Design review of the part built by this model. Coordinates are the model's own, in mm. Face numbers are marked on the shaded views. Give positions to 0.01 mm unless a question says otherwise; leave off trailing zeros. Order: outer loops, then holes, each group sorted by start corner. A loop starts at its lowest first (then second) coordinate and runs counter-clockwise, first axis right, second up. Notation, with made-up numbers: (40.5, 25) -> (66.5, 25) arc R10 ccw to (66.5, 35) -> close; hole circle Ø10 at (84, 77). An arc over 180 degrees is marked (long way). One line per item, written item: value. Start each with the question number.
1) Consider section C-C (y = 4.2). State how many separate pieces and enclosed holes the cut face has, plus the area to 3 significant figures.
2) For pin 1 (1.6 mm diameter, centred on y = 2, z = 9.5, fed in from -X); pin 2 (2.5 mm diameter, centred on y = 2, z = 9.5, fed in from +X); pin 3 (3 mm diameter, centred on x = 76.5, y = 3, fed in from +Z), all flat-tipped, find the tip position at first contact; note any pin that passes through.
3) Wall thickness on line 1 along X through (y, z) = (4.1, -129); line 2 along Z through (x, y) = (119, 1.7); line 3 along Y through (x, z) = (164.5, -63): over which ranges is each line inside the solid? List them lowest first. Write a range as from..to.
4) Consider section D-D (x = 164). State the section outline as (y, z) points.
5) Consider section B-B (z = -161). State the section outline as (x, y) points.
6) The part is to be moulded in two halves that separate along Z. For the marked faces 1 and 2, say which applies: released by +Z, released by -Z, zero draft, split by the parting line, or undercut.
Autodesk Fusion 360 part; units mm, degrees
sketch "Sketch1" plane through (0, 0, 0) normal (0, 1, 0) x (1, 0, 0)
  line L0 (0, 0) -> (230.6, 0)
  line L1 (230.6, 0) -> (230.6, 183)
  line L2 (230.6, 183) -> (0, 183)
  line L3 (0, 183) -> (0, 0)
  dimension "d1" = 230.6
  dimension "d2" = 183
extrude "Extrude1" add sketch "Sketch1" along normal blind 10
sketch "Sketch9" plane through (0, 0, 0) normal (-1, 0, 0) x (0, 0, 1)
  line L0 (-183, 0) -> (0, 0)
  line L1 (0, 0) -> (0, 10)
  line L2 (0, 10) -> (-183, 10)
  line L3 (-183, 10) -> (-183, 0)
  circle A0 centre (11.4881, 10.5) radius 10.5
  line L4 (11.4881, 0) -> (0, 0)
  circle A1 centre (11.4881, 10.5) radius 9
  line L5 (0, 0) -> (1, 0)
  line L6 (1, 0) -> (1, 10)
  line L7 (1, 10) -> (0, 10)
  line L8 (0, 10) -> (0, 0)
  dimension "d69" = 21
  dimension "d70" = 18
  dimension "d94" = 1
extrude "Extrude8" add sketch "Sketch9" against normal up to surface (230.6 mm away) contours L1 L4 L5 L6 L7 L8 | A0 L4 L6 | A0
sketch "Sketch10" plane through (0, 0, 0) normal (0, -1, 0) x (1, 0, 0)
  line L0 (230.6, -183) -> (230.6, 11.4881)
  line L1 (230.6, 11.4881) -> (0, 11.4881)
  line L2 (0, 11.4881) -> (0, -183)
  line L3 (230.6, 0) -> (218.6, 0)
  line L4 (218.6, 0) -> (218.6, 22)
  line L5 (218.6, 22) -> (230.6, 22)
  line L6 (230.6, 22) -> (230.6, 0)
  line L7 (203.6, 0) -> (27, 0)
  line L8 (27, 0) -> (27, 22)
  line L9 (27, 22) -> (203.6, 22)
  line L10 (203.6, 22) -> (203.6, 0)
  line L11 (0, 0) -> (12, 0)
  line L12 (12, 0) -> (12, 22)
  line L13 (12, 22) -> (0, 22)
  line L14 (0, 22) -> (0, 0)
  line L15 (0, -183) -> (230.6, -183)
  dimension "d73" = 22
  dimension "d74" = 12
  dimension "d75" = 12
  dimension "d76" = 15
  dimension "d77" = 15
extrude "Extrude9" cut sketch "Sketch10" against normal through all contours L0 L1 L3 L4 L6 | L1 L4 L5 L6 | L1 L2 L11 L12 L14 | L1 L12 L13 L14 | L1 L7 L8 L10 | L1 L8 L9 L10
sketch "Sketch11" plane through (0, 10, 0) normal (0, 1, 0) x (-1, 0, 0)
  line L0 (0, -183) -> (0, 0)
  line L1 (-1.8, -176) -> (-228.8, -176)
  line L2 (-228.8, -176) -> (-228.8, -1)
  line L3 (-228.8, -1) -> (-1.8, -1)
  line L4 (-1.8, -1) -> (-1.8, -176)
  line L5 (-115.3, -122.9084) -> (-115.3, -50) construction
  line L6 (-230.6, 0) -> (-230.6, -183)
  line L7 (-230.6, -183) -> (0, -183)
  line L8 (-12, 0) -> (-12, 1)
  line L9 (-12, 1) -> (-27, 1)
  line L10 (-27, 1) -> (-27, 0)
  line L11 (-27, 0) -> (-203.6, 0)
  line L12 (-203.6, 0) -> (-203.6, 1)
  line L13 (-203.6, 1) -> (-218.6, 1)
  line L14 (-218.6, 1) -> (-218.6, 0)
  line L15 (-218.6, 0) -> (-230.6, 0)
  line L16 (0, 0) -> (-12, 0)
  dimension "d79" = 227
  dimension "d80" = 175
extrude "Extrude10" cut sketch "Sketch11" against normal blind 2 contours L1 L2 L3 L4
sketch "Sketch12" plane through (0, 8, 0) normal (0, 1, 0) x (-1, 0, 0)
  line L0 (-1.8, -1) -> (-228.8, -1)
  line L1 (-1.8, -176) -> (-1.8, -1)
  line L2 (-6.95, -6.345) -> (-223.65, -6.345)
  line L3 (-223.65, -6.345) -> (-223.65, -181.345)
  line L4 (-223.65, -181.345) -> (-6.95, -181.345)
  line L5 (-6.95, -181.345) -> (-6.95, -6.345)
  line L6 (-10.47, -167.125) -> (-220.13, -167.125)
  line L7 (-220.13, -167.125) -> (-220.13, -9.875)
  line L8 (-220.13, -9.875) -> (-10.47, -9.875)
  line L9 (-10.47, -9.875) -> (-10.47, -167.125)
  line L10 (-85, -88.5) -> (-145, -88.5) construction
  line L11 (-115.3, -115.3819) -> (-115.3, -64.9996) construction
  line L12 (-228.8, -1) -> (-228.8, -176)
  line L13 (-228.8, -176) -> (-1.8, -176)
  dimension "d84" = 175
  dimension "d85" = 216.7
  dimension "d86" = 209.66
  dimension "d87" = 157.25
  dimension "d88" = 3.52
  dimension "d89" = 3.53
extrude "Extrude11" cut sketch "Sketch12" against normal blind 1 contours L2 L3 L5 L13 | L3 L4 L5 L13 | L6 L7 L8 L9
fillet "Fillet1" radius 6 2 edges at (0, 5, -183) (230.6, 5, -183)
sketch "Sketch15" plane through (12, 0, 0) normal (-1, 0, 0) x (0, 0, 1)
  line L0 (0, 10) -> (0, 0)
  line L1 (0, 0) -> (11.4881, 0)
  arc A0 (11.4881, 0) -> (1, 10) centre (11.4881, 10.5) ccw
  circle A1 centre (11.4881, 10.5) radius 11.499
  line L2 (0, 0) -> (6.8002, 0)
  line L3 (1, 10) -> (0, 10)
  circle A2 centre (11.4881, 10.5) radius 9
extrude "Extrude14" add sketch "Sketch15" along normal blind 12 and the other way blind 218.6 contours L0 L1 A1 L2
sketch "Sketch13" plane through (0, 0, 0) normal (-1, 0, 0) x (0, 0, 1)
  line L0 (-177, 10) -> (-177, 0)
  line L1 (-177, 0) -> (6.8002, 0)
  line L2 (0, 10) -> (-177, 10)
  line L3 (-183, 5.4) -> (22, 5.4)
  line L4 (22, 5.4) -> (22, 23.4)
  line L5 (22, 23.4) -> (-183, 23.4)
  line L6 (-183, 23.4) -> (-183, 5.4)
  arc A0 (0, 10) -> (6.8002, 0) centre (11.4881, 10.5) ccw
  dimension "d95" = 4.6
  dimension "d96" = 6
  dimension "d97" = 205
  dimension "d98" = 18
extrude "Extrude12" cut sketch "Sketch13" against normal through all contours L0 L2 L3 A0 | L0 L2 L3 L4 L5 L6 A0
sketch "Sketch14" plane through (0, 5.4, 0) normal (0, 1, 0) x (-1, 0, 0)
  arc A0 (-6, -183) -> (0, -177) centre (-6, -177) ccw
  line L0 (0, -177) -> (0, 1.182)
  line L1 (-12, 1.182) -> (-12, 4.0726)
  line L2 (-12, 4.0726) -> (-27, 4.0726)
  line L3 (-27, 4.0726) -> (-27, 1.182)
  line L4 (-203.6, 1.182) -> (-203.6, 4.0726)
  line L5 (-203.6, 4.0726) -> (-218.6, 4.0726)
  line L6 (-218.6, 4.0726) -> (-218.6, 1.182)
  line L7 (-230.6, 1.182) -> (-230.6, -177)
  arc A1 (-230.6, -177) -> (-224.6, -183) centre (-224.6, -177) ccw
  line L8 (-224.6, -183) -> (-6, -183)
  line L9 (-2, -177) -> (-2, -2)
  line L10 (-2, -2) -> (-14, -2)
  line L11 (-14, -2) -> (-14, 2.0726)
  line L12 (-14, 2.0726) -> (-25, 2.0726)
  line L13 (-25, 2.0726) -> (-25, -2)
  line L14 (-25, -2) -> (-205.6, -2)
  line L15 (-205.6, -2) -> (-205.6, 2.0726)
  line L16 (-205.6, 2.0726) -> (-216.6, 2.0726)
  line L17 (-216.6, 2.0726) -> (-216.6, -2)
  line L18 (-216.6, -2) -> (-228.6, -2)
  line L19 (-228.6, -2) -> (-228.6, -177)
  arc A2 (-228.6, -177) -> (-224.6, -181) centre (-224.6, -177) ccw
  line L20 (-224.6, -181) -> (-6, -181)
  arc A3 (-6, -181) -> (-2, -177) centre (-6, -177) ccw
  line L21 (-14, 2.0726) -> (-25, 2.0726)
  line L22 (-25, 2.0726) -> (-25, 11.5726)
  line L23 (-25, 11.5726) -> (-14, 11.5726)
  line L24 (-14, 11.5726) -> (-14, 2.0726)
  line L25 (-205.6, 2.0726) -> (-216.6, 2.0726)
  line L26 (-216.6, 2.0726) -> (-216.6, 11.5726)
  line L27 (-216.6, 11.5726) -> (-205.6, 11.5726)
  line L28 (-205.6, 11.5726) -> (-205.6, 2.0726)
  line L29 (-27, 1.182) -> (-203.6, 1.182)
  line L30 (-218.6, 1.182) -> (-230.6, 1.182)
  line L31 (0, 1.182) -> (-12, 1.182)
  dimension "d101" = 9.5
  dimension "d102" = 9.5
extrude "Extrude13" cut sketch "Sketch14" against normal blind 3.9 contours L2 L12 L21 L22 L24 | L2 L22 L23 L24 | L9 L10 L11 L12 L13 L14 L15 L16 L17 L18 L19 A2 L20 A3 L21 L25 | L5 L26 L27 L28 | L5 L16 L25 L26 L28
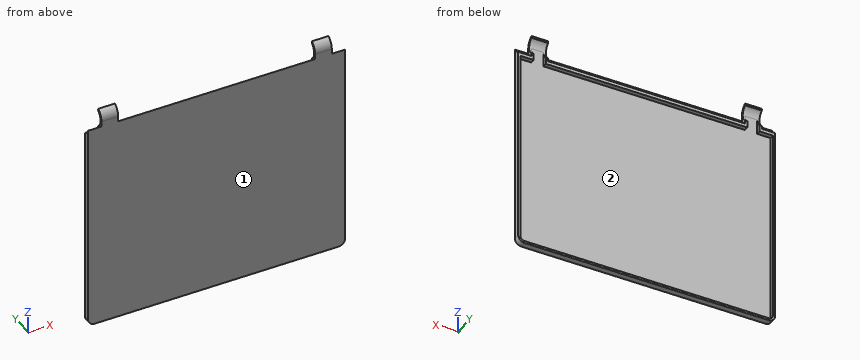
Checked values:
1. separate pieces: 4
1. enclosed holes: 0
1. area: 2,060 mm^2
2. pin 1: stops at x = 12
2. pin 2: stops at x = 218.6
2. pin 3: stops at z = 4.33
3. line 1: x = 0..2, 228.6..230.6
3. line 2: z = -183..-181, -2..4.09
3. line 3: y = 0..1.5
4. outline: (0, -183) -> (5.4, -183) -> (5.4, -181) -> (1.5, -181) -> (1.5, -2) -> (5.4, -2) -> (5.4, 1.18) arc R11.5 cw to (0, 6.8) -> close
5. outline: (0, 0) -> (230.6, 0) -> (230.6, 5.4) -> (228.6, 5.4) -> (228.6, 1.5) -> (2, 1.5) -> (2, 5.4) -> (0, 5.4) -> close
6. face 1: zero draft
6. face 2: undercut
